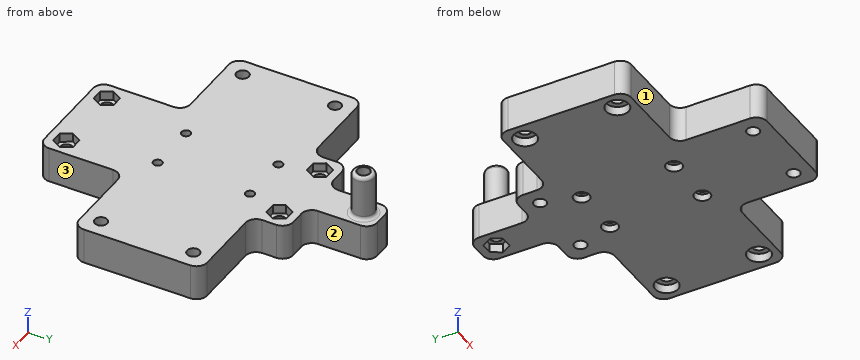
```python
from build123d import *

# Parameters (mm, degrees)
SKETCH_2_W          = 25
SKETCH_2_H          = 25
SKETCH_2_R          = 1.75
SKETCH_2_H_2        = 11
SKETCH_2_W_2        = 30
SKETCH_2_R_2        = 1.25
SKETCH_2_H_3        = 24
SKETCH_2_W_3        = 10
SKETCH_2_H_4        = 10
SKETCH_2_H_5        = 18
EXTRUDE_1_DEPTH     = 10
SKETCH_4_R          = 3.2
CUT_EXTRUDE_2_DEPTH = 2.5
SKETCH_5_R          = 2.2
CUT_EXTRUDE_3_DEPTH = 2
FILLET_2_R          = 3
CUT_EXTRUDE_4_DEPTH = 2.5
CUT_EXTRUDE_5_DEPTH = 2.5
SKETCH_8_R          = 3
SKETCH_8_R_2        = 1.75
EXTRUDE_2_DEPTH     = 12.5
FILLET_3_R          = 1


with BuildPart() as part:
    # ｽｹｯﾁ2 → ﾎﾞｽ - 押し出し1 (new body)
    # profile 1 of 11: a face of its own
    with BuildSketch(Plane.XY):
        with Locations((-27.5, 5.5)):
            Rectangle(SKETCH_2_W, SKETCH_2_H)
        with Locations((-35, 13)):
            Circle(SKETCH_2_R, mode=Mode.SUBTRACT)
    # profile 2 of 11: a face of its own
    with BuildSketch(Plane.XY):
        with Locations((-27.5, -12.5)):
            Rectangle(SKETCH_2_W, SKETCH_2_H_2)
        with Locations((-35, -13)):
            Circle(SKETCH_2_R, mode=Mode.SUBTRACT)
    # profile 3 of 11: a face of its own
    with BuildSketch(Plane.XY):
        with Locations((0, -12.5)):
            Rectangle(SKETCH_2_W_2, SKETCH_2_H_2)
        with Locations((-7, -13)):
            Circle(SKETCH_2_R_2, mode=Mode.SUBTRACT)
        with Locations((7, -13)):
            Circle(SKETCH_2_R_2, mode=Mode.SUBTRACT)
    # profile 4 of 11: a face of its own
    with BuildSketch(Plane.XY):
        Polygon((15, 18), (5, 18), (-5, 18), (-15, 18), (-15, -7), (15, -7), align=None)
        with Locations((-7, 13)):
            Circle(SKETCH_2_R_2, mode=Mode.SUBTRACT)
        with Locations((7, 13)):
            Circle(SKETCH_2_R_2, mode=Mode.SUBTRACT)
    # profile 5 of 11: a face of its own
    with BuildSketch(Plane.XY):
        with Locations((27.5, 5.5)):
            Rectangle(SKETCH_2_W, SKETCH_2_H)
        with Locations((35, 13)):
            Circle(SKETCH_2_R, mode=Mode.SUBTRACT)
    # profile 6 of 11: a face of its own
    with BuildSketch(Plane.XY):
        with Locations((27.5, -12.5)):
            Rectangle(SKETCH_2_W, SKETCH_2_H_2)
        with Locations((35, -13)):
            Circle(SKETCH_2_R, mode=Mode.SUBTRACT)
    # profile 7 of 11: a face of its own
    with BuildSketch(Plane.XY):
        with Locations((0, -30)):
            Rectangle(SKETCH_2_W_2, SKETCH_2_H_3)
        with Locations((-10, -37)):
            Circle(SKETCH_2_R, mode=Mode.SUBTRACT)
        with Locations((10, -37)):
            Circle(SKETCH_2_R, mode=Mode.SUBTRACT)
    # profile 8 of 11: a face of its own
    with BuildSketch(Plane.XY):
        with Locations((-10, 23)):
            Rectangle(SKETCH_2_W_3, SKETCH_2_H_4)
        with Locations((-10, 23)):
            Circle(SKETCH_2_R, mode=Mode.SUBTRACT)
    # profile 9 of 11: a face of its own
    with BuildSketch(Plane.XY):
        with Locations((0, 23)):
            Rectangle(SKETCH_2_W_3, SKETCH_2_H_4)
    # profile 10 of 11: a face of its own
    with BuildSketch(Plane.XY):
        with Locations((10, 23)):
            Rectangle(SKETCH_2_W_3, SKETCH_2_H_4)
        with Locations((10, 23)):
            Circle(SKETCH_2_R, mode=Mode.SUBTRACT)
    # profile 11 of 11: a face of its own
    with BuildSketch(Plane.XY):
        with Locations((0, 37)):
            Rectangle(SKETCH_2_W_3, SKETCH_2_H_5)
        with Locations((0, 41)):
            Circle(SKETCH_2_R, mode=Mode.SUBTRACT)
    extrude(amount=EXTRUDE_1_DEPTH)

    # ｽｹｯﾁ4 → ｶｯﾄ - 押し出し2 (cut)
    with BuildSketch(Plane(origin=(0, 0, 0), x_dir=(-1, 0, 0), z_dir=(0, 0, -1))):
        with Locations((-35, 13)):
            Circle(SKETCH_4_R)
        with Locations(Location((35, 13, 0), (0, 0, 180))):
            Circle(SKETCH_4_R)
        with Locations((35, -13)):
            Circle(SKETCH_4_R)
        with Locations(Location((-35, -13, 0), (0, 0, 180))):
            Circle(SKETCH_4_R)
    extrude(amount=-CUT_EXTRUDE_2_DEPTH, mode=Mode.SUBTRACT)

    # ｽｹｯﾁ5 → ｶｯﾄ - 押し出し3 (cut)
    with BuildSketch(Plane(origin=(0, 0, 0), x_dir=(-1, 0, 0), z_dir=(0, 0, -1))):
        with Locations((-7, 13)):
            Circle(SKETCH_5_R)
        with Locations(Location((7, 13, 0), (0, 0, 180))):
            Circle(SKETCH_5_R)
        with Locations((7, -13)):
            Circle(SKETCH_5_R)
        with Locations(Location((-7, -13, 0), (0, 0, 180))):
            Circle(SKETCH_5_R)
    extrude(amount=-CUT_EXTRUDE_3_DEPTH, mode=Mode.SUBTRACT)

    # ﾌｨﾚｯﾄ2
    fillet_2_edges = [part.edges().sort_by_distance(p)[0] for p in [
        (15, -18, 5),
        (15, -42, 5),
        (-15, -42, 5),
        (-15, -18, 5),
        (-40, -18, 5),
        (-40, 18, 5),
        (-15, 18, 5),
        (-15, 28, 5),
        (-5, 28, 5),
        (-5, 46, 5),
        (5, 46, 5),
        (5, 28, 5),
        (15, 28, 5),
        (15, 18, 5),
        (40, 18, 5),
        (40, -18, 5),
    ]]
    fillet(fillet_2_edges, radius=FILLET_2_R)

    # ｽｹｯﾁ6 → ｶｯﾄ - 押し出し4 (cut)
    with BuildSketch(Plane(origin=(0, 0, 0), x_dir=(-1, 0, 0), z_dir=(0, 0, -1))):
        Polygon((3.233161507, 41), (1.616580754, 43.8), (-1.616580754, 43.8), (-3.233161507, 41), (-1.616580754, 38.2), (1.616580754, 38.2), align=None)
    extrude(amount=-CUT_EXTRUDE_4_DEPTH, mode=Mode.SUBTRACT)

    # ｽｹｯﾁ7 → ｶｯﾄ - 押し出し5 (cut)
    with BuildSketch(Plane.XY.offset(10)):
        Polygon((-6.766838493, 23), (-8.383419246, 25.8), (-11.616580754, 25.8), (-13.233161507, 23), (-11.616580754, 20.2), (-8.383419246, 20.2), align=None)
        Polygon((8.383419246, 20.2), (6.766838493, 23), (8.383419246, 25.8), (11.616580754, 25.8), (13.233161507, 23), (11.616580754, 20.2), align=None)
        Polygon((8.383419246, -39.8), (6.766838493, -37), (8.383419246, -34.2), (11.616580754, -34.2), (13.233161507, -37), (11.616580754, -39.8), align=None)
        Polygon((-6.766838493, -37), (-8.383419246, -34.2), (-11.616580754, -34.2), (-13.233161507, -37), (-11.616580754, -39.8), (-8.383419246, -39.8), align=None)
    extrude(amount=-CUT_EXTRUDE_5_DEPTH, mode=Mode.SUBTRACT)

    # ｽｹｯﾁ8 → ﾎﾞｽ - 押し出し2 (add)
    with BuildSketch(Plane.XY.offset(10)):
        with Locations((0, 41)):
            Circle(SKETCH_8_R)
        with Locations(Location((0, 41, 0), (0, 0, 180))):
            Circle(SKETCH_8_R_2, mode=Mode.SUBTRACT)
    extrude(amount=EXTRUDE_2_DEPTH)

    # ﾌｨﾚｯﾄ3
    fillet_3_edges = [part.edges().sort_by_distance(p)[0] for p in [
        (-3, 41, 22.5),
        (-3, 41, 10),
    ]]
    fillet(fillet_3_edges, radius=FILLET_3_R)


solid = part.part
```
For this review, take the finished solid that the model builds, in its own axes (mm). Face numbers are marked on the shaded views. A direction names the side the tool comes from. Round coordinates to 2 decimals unless told otherwise and drop trailing zeros. Write each loop counter-clockwise with the first axis right and the second up, starting at its lowest first coordinate (ties: lowest second). Pieces come first, ordered by that corner, then holes. Notation, with made-up numbers: (68, -35) - (122, -35) arc R26 cw to (122, -4) - close; hole circle Ø10 at (72, 33). An arc over 180 degrees is marked (long way). Put each result on its own line as item: value.
Q1. Insertion check: pin 1 Ø1.2 at (x, z) = (-10.5, 9) entering from +Y; pin 2 Ø1 at (x, z) = (28, 9) entering from +Y; pin 3 Ø8.5 at (x, y) = (35, 13) entering from +Z; pin 4 Ø7 at (x, y) = (-35.5, 12) entering from -Z. Each pin has a flat end and moves straight along its axis. Give the tip position at first contact, or say it passes through.
Solved:
pin 1: stops at y = 28
pin 2: stops at y = 18
pin 3: stops at z = 10
pin 4: stops at z = 0
Q2. Machinability: for the marked faces 1, 2 and 3, which of the approach directions +Z, -Z, +X, -X, +Y, -Y give a long, thin tool a straight path to every point of the face, cutting with its end or side? Answer none if there is none.
Solved:
face 1: +Z, -Z, -X, -Y
face 2: +Z, -Z, +X, +Y
face 3: +Z, -Z, +X, -Y
Q3. Wall thickness on probe 1 along X at (y, z) = (-13, 8.25); probe 2 along Y at (x, z) = (-35, 1.9); probe 3 along Y at (x, z) = (-10, 3): over which ranges is each line inside the solid? List them lowest first.
Solved:
probe 1: x = -40 to -36.75, -33.25 to -8.25, -5.75 to 5.75, 8.25 to 33.25, 36.75 to 40
probe 2: y = -18 to -16.2, -9.8 to 9.8, 16.2 to 18
probe 3: y = -42 to -38.75, -35.25 to 21.25, 24.75 to 28
Q4. We need section A-A (y = -13). Count the separate pieces of the cut face and the enclosed holes in it, and give its area (3 significant figures).
Solved:
separate pieces: 5
enclosed holes: 0
area: 658 mm2
Q5. We need section B-B (z = 15.5). Give the boundary of the cut face in (x, y).
Solved:
outline: circle Ø6 at (0, 41); hole circle Ø3.5 at (0, 41)
Q6. We need section C-C (y = -30.5). Give the boundary of the cut face in (x, z).
Solved:
outline: (-15, 0) - (15, 0) - (15, 10) - (-15, 10) - close
